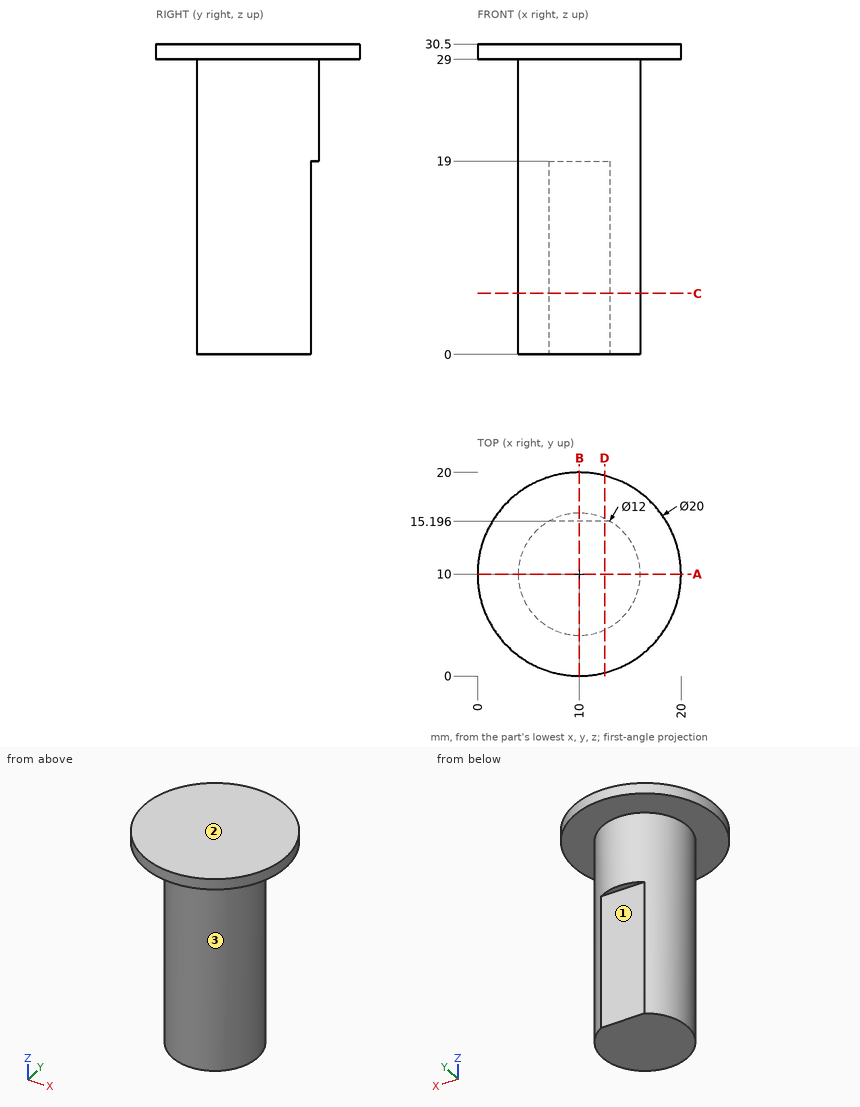
Design review of the part shown in the three views and the two pictorial views. Dimensions are in mm from the part's minimum x, y and z. A direction names the side the tool comes from. Round coordinates to 2 decimals unless told otherwise and drop trailing zeros. Order: outer loops, then holes, each group sorted by start corner. A loop starts at its lowest first (then second) coordinate and runs counter-clockwise, first axis right, second up.
Q1. We need section B-B, the plane x = 10. Give the boundary of the cut face in (y, z).
Findings below:
outline: (0, 29) - (4, 29) - (4, 0) - (15.2, 0) - (15.2, 19) - (16, 19) - (16, 29) - (20, 29) - (20, 30.5) - (0, 30.5) - close
Q2. Machinability: for the marked faces 1, 2 and 3, which of the approach directions +Z, -Z, +X, -X, +Y, -Y give a long, thin tool a straight path to every point of the face, cutting with its end or side? Answer none if there is none.
Findings below:
face 1: -Z, +X, -X, +Y
face 2: +Z, +X, -X, +Y, -Y
face 3: -Z
Q3. We need section D-D, the plane x = 12.5. Give the boundary of the cut face in (y, z).
Findings below:
outline: (0.32, 29) - (4.55, 29) - (4.55, 0) - (15.2, 0) - (15.2, 19) - (15.45, 19) - (15.45, 29) - (19.68, 29) - (19.68, 30.5) - (0.32, 30.5) - close
Q4. Insertion check: P1, Ø1.5, axis at x = 5.5, z = 13.5, coming from the -Y side; P2, Ø1.5, axis at y = 15, z = 17.5, coming from the -X side (1 decimal); P3, Ø12, axis at y = 14, z = 4, coming from the +X side; P4, Ø2, axis at y = 16.5, z = 14, coming from the -X side. Each pin has a flat end and moves straight along its axis. Give the tip position at first contact, or say it passes through.
Findings below:
P1: stops at y = 5.32
P2: stops at x = 5.8
P3: stops at x = 16
P4: passes through
Q5. We need section C-C, the plane z = 6. Give the boundary of the cut face in (x, y).
Findings below:
outline: (7, 15.2) arc R6 ccw (long way) to (13, 15.2) - close
Q6. Wall thickness on line 1 (Z direction, x = 6.25, y = 16); line 2 (Z direction, x = 10.25, y = 15.75); line 3 (Y direction, x = 12.5, z = 7): over which ranges is each line inside the solid? List them lowest first.
Findings below:
line 1: z = 29 to 30.5
line 2: z = 19 to 30.5
line 3: y = 4.55 to 15.2
Q7. We need section A-A, the plane y = 10. Give the boundary of the cut face in (x, z), plus the area to 3 significant figures.
Findings below:
outline: (0, 29) - (4, 29) - (4, 0) - (16, 0) - (16, 29) - (20, 29) - (20, 30.5) - (0, 30.5) - close
area: 378 mm2
